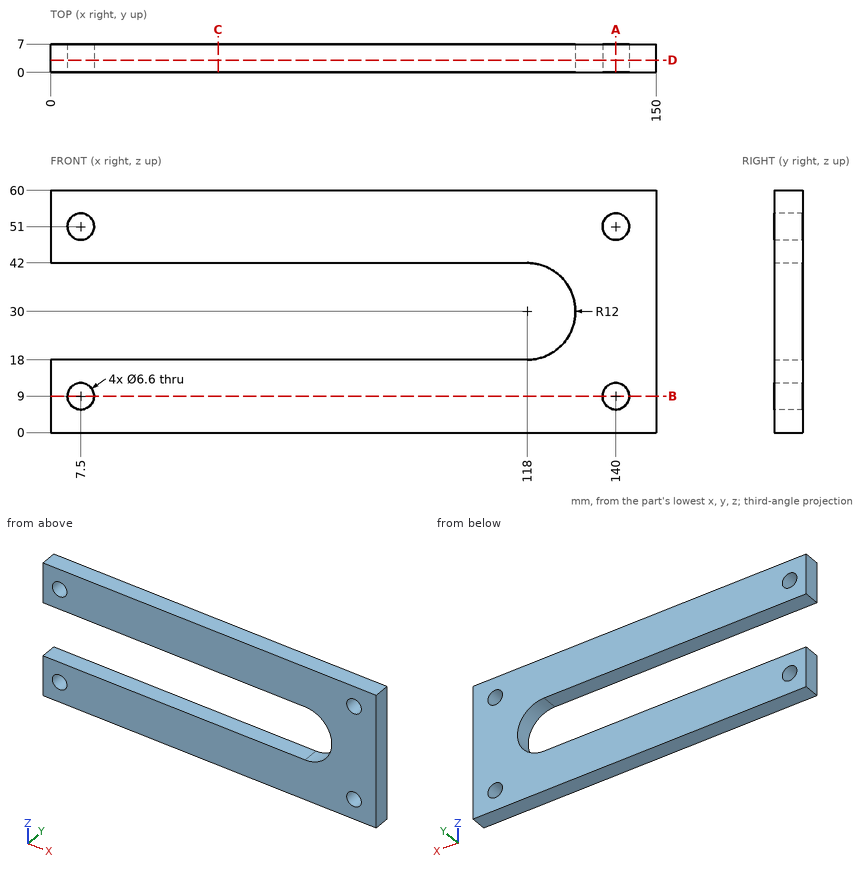
Geometry check sheet. Reference: drawing and pictorial views, mm from the part's lowest x, y, z. Coordinates: 2 decimals unless noted, no trailing zeros. Order: outer loops, then holes, each group sorted by start corner. A loop starts at its lowest first (then second) coordinate and runs counter-clockwise, first axis right, second up. Notation, with made-up numbers: (24.25, 13.25) - (61.25, 13.25) arc R16 cw to (61.25, 34.25) - close; hole circle Ø8 at (50.25, -36.5). An arc over 180 degrees is marked (long way). Answer in a Markdown table with one row per item. Add a question column.
1) Cross-section at D-D, the plane y = 3. Record the cut outline in (x, z), then the cut area to 3 significant figures.
2) Cross-section at B-B, the plane z = 9. Record the cut outline in (x, y), then the cut area to 3 significant figures.
3) Cross-section at A-A, the plane x = 140. Record the cut outline in (y, z).
4) Gauge pin test, flat end, axial feed: P1, Ø8.5, axis at x = 7.5, z = 51, coming from the +Y side. Record the tip position at first contact, or that the pin passes through.
5) Cross-section at C-C, the plane x = 41.5. Record the cut outline in (y, z).
6) Material ranges on line 1 along Z through (x, y) = (140, 2.5); line 2 along X through (y, z) = (5.5, 51); line 3 along Z through (x, y) = (85.5, 6.25), recorded low to high. Write a range as [from, to].
Check result:
| question | item | result |
|---|---|---|
| 1 | outline | (0, 0) - (150, 0) - (150, 60) - (0, 60) - (0, 42) - (118, 42) arc R12 cw to (118, 18) - (0, 18) - close; hole circle Ø6.6 at (7.5, 9); hole circle Ø6.6 at (7.5, 51); hole circle Ø6.6 at (140, 9); hole circle Ø6.6 at (140, 51) |
| 1 | area | 5,800 mm² |
| 2 | outline | (0, 0) - (4.2, 0) - (4.2, 7) - (0, 7) - close; (10.8, 0) - (136.7, 0) - (136.7, 7) - (10.8, 7) - close; (143.3, 0) - (150, 0) - (150, 7) - (143.3, 7) - close |
| 2 | area | 958 mm² |
| 3 | outline | (0, 0) - (7, 0) - (7, 5.7) - (0, 5.7) - close; (0, 12.3) - (7, 12.3) - (7, 47.7) - (0, 47.7) - close; (0, 54.3) - (7, 54.3) - (7, 60) - (0, 60) - close |
| 4 | P1 | stops at y = 7 |
| 5 | outline | (0, 0) - (7, 0) - (7, 18) - (0, 18) - close; (0, 42) - (7, 42) - (7, 60) - (0, 60) - close |
| 6 | line 1 | z = [0, 5.7], [12.3, 47.7], [54.3, 60] |
| 6 | line 2 | x = [0, 4.2], [10.8, 136.7], [143.3, 150] |
| 6 | line 3 | z = [0, 18], [42, 60] |
